Geometry: final body of the model. Coordinates: model frame, mm. Give positions to 0.01 mm unless a question says otherwise; leave off trailing zeros. Write each loop counter-clockwise with the first axis right and the second up, starting at its lowest first coordinate (ties: lowest second). Pieces come first, ordered by that corner, then holes. Notation, with made-up numbers: M 23,74 L 39,74 A24 ccw 39,86 Z; hole C 66.5,30.5 d2. An arc over 180 degrees is marked long. Use a Markdown table: item, result. Add a question column.
1) Line query: line 1 (Z direction, x = 0, y = 4.4); line 2 (Z direction, x = -0.75, y = 2.35). Output: solid intervals per line, ascending.
2) Draft query along X for faces 1 (the cylindrical face through (3.937, 3.458, -1.24)), 2 (the flat face through (2, 4.763, 2)), 3 (the cylindrical face through (-1.97, 4.18, 0.62)). Return one class per face: +X half, -X half, draft (parallel to the pull), parting line (faces both ways), or undercut.
3) Pin query (flat end, axial travel): pin 1 (1.5 mm diameter, centred on y = 3, z = -1.5, fed in from -X); pin 2 (2.5 mm diameter, centred on x = 0, z = 0, fed in from -Y); pin 3 (1 mm diameter, centred on x = 2, y = 4, fed in from +Z). Return the tip coordinate at first contact, or that it passes through.
4) Section A-A on y = 4.15. Return the cut outline in (x, z) (1 decimal), then the cut area to 3 significant figures.
```python
from build123d import *

# Parameters (mm, degrees)
SKETCH2_R          = 2.06375
CUT_EXTRUDE1_DEPTH = 7.404538696


with BuildPart() as part:
    # Sketch1 → Revolve1 (revolve)
    with BuildSketch(Plane.XY):
        with BuildLine():
            Line((4.1275, 0), (4.1275, 4.7625))
            Line((4.1275, 4.7625), (0, 4.7625))
            Line((0, 4.7625), (0, 4.1275))
            ThreePointArc((0, 4.1275), (2.918583239, 2.918583239), (4.1275, 0))
        make_face()
    revolve(axis=Axis((0, -74.223969944, 0), (0, 1, 0)))

    # Fillet1: read off the stored shape, not the designer's step
    # Fillet1 outline → Fillet1 (revolve, cut)
    with BuildSketch(Plane.XY):
        with BuildLine():
            Line((3.429894366, 2.127048943), (3.7465, 2.127049042))
            ThreePointArc((3.7465, 2.127049042), (3.567044036, 2.17195894), (3.429894366, 2.296101236))
            Line((3.429894366, 2.296101236), (3.429894366, 2.127048943))
        make_face()
        with BuildLine():
            Line((3.7465, 2.127049042), (4.1275, 2.127048943))
            Line((4.1275, 2.127048943), (4.1275, 2.508049043))
            ThreePointArc((4.1275, 2.508049043), (4.015907684, 2.238641359), (3.7465, 2.127049042))
        make_face()
        with BuildLine():
            ThreePointArc((3.7465, 4.7625), (4.015907684, 4.650907684), (4.1275, 4.3815))
            Line((4.1275, 4.3815), (4.1275, 4.7625))
            Line((4.1275, 4.7625), (3.7465, 4.7625))
        make_face()
    revolve(axis=Axis((0, 0, 0), (0, 1, 0)), mode=Mode.SUBTRACT)

    # Fillet1 2 outline → Fillet1 2 (revolve, cut)
    with BuildSketch(Plane.XY):
        with BuildLine():
            ThreePointArc((3.53721911, 2.127048947), (3.977192988, 1.103717438), (4.1275, -4e-09))
            Line((4.1275, -4e-09), (4.1275, 2.127048943))
            Line((4.1275, 2.127048943), (3.7465, 2.127049042))
            Line((3.7465, 2.127049042), (3.53721911, 2.127048947))
        make_face()
    revolve(axis=Axis((0, 0, 0), (0, 1, 0)), mode=Mode.SUBTRACT)

    # Sketch2 → Cut-Extrude1 (cut, through all)
    with BuildSketch(Plane(origin=(0, 4.7625, 0), x_dir=(1, 0, 0), z_dir=(0, 1, 0))):
        with Locations(Location((0, 0, 0), (0, 0, 180))):
            Circle(SKETCH2_R)
    extrude(amount=-CUT_EXTRUDE1_DEPTH, mode=Mode.SUBTRACT)


solid = part.part
```
Found:
| question | item | result |
|---|---|---|
| 1 | line 1 | -4.13 to -2.06, 2.06 to 4.13 |
| 1 | line 2 | -4.02 to -3.31, 3.31 to 4.02 |
| 2 | face 1 | parting line |
| 2 | face 2 | draft |
| 2 | face 3 | undercut |
| 3 | pin 1 | x = -4.06 |
| 3 | pin 2 | through |
| 3 | pin 3 | z = 3.85 |
| 4 | outline | C 0,0 d8.3; hole C 0,0 d4.1 |
| 4 | area | 40.1 mm² |
